from build123d import *

# Parameters (mm, degrees)
SKETCH1_R           = 22.5
BOSS_EXTRUDE1_DEPTH = 25
SKETCH2_R           = 12.5
CUT_EXTRUDE1_DEPTH  = 10
FILLET1_R           = 5
SKETCH3_R           = 1.5
CUT_EXTRUDE2_DEPTH  = 41.466035196
CUT_EXTRUDE3_DEPTH  = 41.466035196


with BuildPart() as part:
    # Sketch1 → Boss-Extrude1 (new body)
    with BuildSketch(Plane(origin=(0, 0, 0), x_dir=(0, 0, -1), z_dir=(1, 0, 0))):
        Circle(SKETCH1_R)
    extrude(amount=BOSS_EXTRUDE1_DEPTH)

    # Sketch2 → Cut-Extrude1 (cut)
    with BuildSketch(Plane(origin=(25, 0, 0), x_dir=(0, 0, -1), z_dir=(1, 0, 0))):
        Circle(SKETCH2_R)
    extrude(amount=-CUT_EXTRUDE1_DEPTH, mode=Mode.SUBTRACT)

    # Fillet1
    fillet1_edges = [part.edges().sort_by_distance(p)[0] for p in [
        (0, 0, 22.5),
        (25, 0, 22.5),
    ]]
    fillet(fillet1_edges, radius=FILLET1_R)

    # Sketch3 → Cut-Extrude2 (cut, through all)
    with BuildSketch(Plane.ZY):
        Circle(SKETCH3_R)
    extrude(amount=-CUT_EXTRUDE2_DEPTH, mode=Mode.SUBTRACT)

    # Sketch4 → Cut-Extrude3 (cut, through all)
    with BuildSketch(Plane.ZY):
        with BuildLine():
            Line((-2.56, -1.92), (2.56, -1.92))
            ThreePointArc((2.56, -1.92), (3.2, 0), (2.56, 1.92))
            Line((2.56, 1.92), (-2.56, 1.92))
            ThreePointArc((-2.56, 1.92), (-3.2, 0), (-2.56, -1.92))
        make_face()
    extrude(amount=-CUT_EXTRUDE3_DEPTH, mode=Mode.SUBTRACT)


solid = part.part
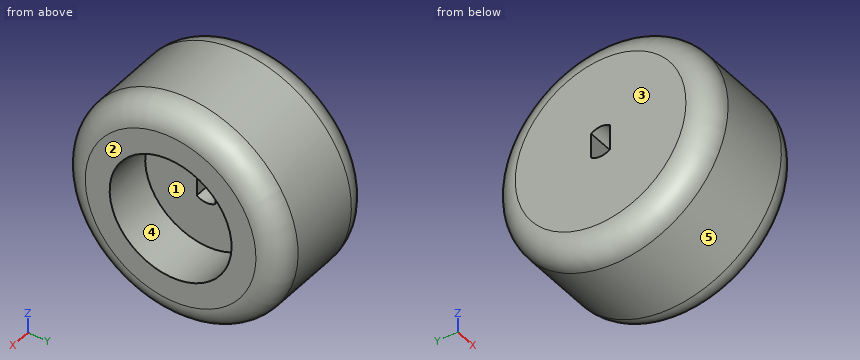
Design review of the part built by this model. Coordinates are the model's own, in mm. Face numbers are marked on the shaded views. A direction names the side the tool comes from. Coordinates: 2 decimals unless noted, no trailing zeros. Loops run counter-clockwise (first coordinate to the right, second up) from the corner with the lowest first, then second, coordinate; pieces in that order, holes last. Notation, with made-up numbers: (-30.75, 30) -> (9.25, 30) arc R14 ccw to (9.25, 45) -> close; hole circle Ø8 at (8, -26.5). An arc over 180 degrees is marked (long way). Use a Markdown table: item, result. Add a question column.
Item 1: We need section C-C, the plane x = 3.25. Write out the cut boundary in (y, z), and give its area (3 significant figures).
Item 2: Clearance check with flat-ended pins moving along their axes: P1, Ø12, axis at x = 13, z = -15, coming from the +Y side; P2, Ø8, axis at x = 15, y = 3.5, coming from the +Z side; P3, Ø5.5, axis at x = 7, z = 1, coming from the -Y side; P4, Ø1.5, axis at x = 2.5, y = -7, coming from the -Z side. State where each tip first meets the part, or that it passes through.
Item 3: We need section D-D, the plane x = 18.75. Write out the cut boundary in (y, z), and give its area (3 significant figures).
Item 4: Wall thickness on L1, parallel to Y at x = 19.25, z = 0; L2, parallel to Y at x = 18.75, z = 3; L3, parallel to X at y = -6.5, z = 3: over which ranges is each line inside the solid? List them lowest first. Write a range as from..to.
Item 5: Machinability: for the marked faces 1 and 2, which of the approach directions +Z, -Z, +X, -X, +Y, -Y give a long, thin tool a straight path to every point of the face, cutting with its end or side? Answer none if there is none.
Item 6: We need section A-A, the plane z = 0. Write out the cut boundary in (x, y), and give its area (3 significant figures).
Item 7: We need section B-B, the plane y = 0. Write out the cut boundary in (x, z).
Item 8: The part is to be moulded in two halves that separate along Y. For the marked faces 3, 4 and 5, say which applies: +Y half, -Y half, draft (parallel to the pull), parting line (faces both ways), or undercut.
Numbers:
| question | item | result |
|---|---|---|
| 1 | outline | circle Ø44.37 at (0, 0); hole (-1.92, -2.56) arc R3.2 ccw to (1.92, -2.56) -> (1.92, 2.56) arc R3.2 ccw to (-1.92, 2.56) -> close |
| 1 | area | 1,520 mm^2 |
| 2 | P1 | stops at y = 20.62 |
| 2 | P2 | stops at z = 22.5 |
| 2 | P3 | stops at y = -22.5 |
| 2 | P4 | stops at z = -21.13 |
| 3 | outline | circle Ø45 at (0, 0); hole circle Ø25 at (0, 0) |
| 3 | area | 1,100 mm^2 |
| 4 | L1 | y = -22.5..-12.5, 12.5..22.5 |
| 4 | L2 | y = -22.3..-12.13, 12.13..22.3 |
| 4 | L3 | x = 0..15 |
| 5 | face 1 | +X |
| 5 | face 2 | +Z, -Z, +X, +Y, -Y |
| 6 | outline | (0, -17.5) arc R5 ccw to (5, -22.5) -> (20, -22.5) arc R5 ccw to (25, -17.5) -> (25, -12.5) -> (15, -12.5) -> (15, -1.92) -> (0, -1.92) -> close; (0, 1.92) -> (15, 1.92) -> (15, 12.5) -> (25, 12.5) -> (25, 17.5) arc R5 ccw to (20, 22.5) -> (5, 22.5) arc R5 ccw to (0, 17.5) -> close |
| 6 | area | 796 mm^2 |
| 7 | outline | (0, -17.5) arc R5 ccw to (5, -22.5) -> (20, -22.5) arc R5 ccw to (25, -17.5) -> (25, -12.5) -> (15, -12.5) -> (15, -3.2) -> (0, -3.2) -> close; (0, 3.2) -> (15, 3.2) -> (15, 12.5) -> (25, 12.5) -> (25, 17.5) arc R5 ccw to (20, 22.5) -> (5, 22.5) arc R5 ccw to (0, 17.5) -> close |
| 8 | face 3 | draft |
| 8 | face 4 | undercut |
| 8 | face 5 | parting line |
